Can you work these out from the drawing? Everything is in mm from the part's minimum corner. A direction names the side the tool comes from. Round coordinates to 2 decimals unless told otherwise and drop trailing zeros. Write each loop counter-clockwise with the first axis right and the second up, starting at its lowest first coordinate (ties: lowest second). Pieces come first, ordered by that corner, then holes. Notation, with made-up numbers: (-34.5, 43.5) -> (-27.5, 43.5) arc R29 ccw to (-27.5, 74.5) -> close; hole circle Ø11 at (35.25, 40.25). An arc over 180 degrees is marked (long way). Put each result on its own line as item: value. Start each with the question number.
1. Suppose I cut it at C-C (y = 6.5). Please give me the cut outline in (x, z), then the cut area to 3 significant figures.
2. Suppose I cut it at D-D (x = 11.5). Please give me the cut outline in (y, z).
3. Which directions (+Z, -Z, +X, -X, +Y, -Y) give clear straight access to the entire face, cutting with the end or side of a thin tool? Please do the marked faces 1 and 2.
4. I need wall thicknesses on probe 1 along Z at (x, y) = (16.7, 4.75); probe 2 along Z at (x, y) = (9, 17.25). Which ranges of each line are inside material? Lowest first, please. Write a range as from..to.
5. Suppose I cut it at A-A (y = 13.5). Please give me the cut outline in (x, z).
6. Suppose I cut it at B-B (z = 23.3). Please give me the cut outline in (x, y).
7. We'd pull the mould along X, two halves only. Please class the marked faces 3, 4, 5 and 6: +X half, -X half, draft (parallel to the pull), parting line (faces both ways), or undercut.
8. For pin 1 (6 mm diameter, centred on x = 16.5, z = 11.5, fed in from +Y); pin 2 (9 mm diameter, centred on x = 12, y = 12, fed in from +Z); pin 3 (4 mm diameter, centred on x = 6, z = 10, fed in from +Y), each with a flat end and sliding along its axis, tell me the tip position at first contact or that it passes through.
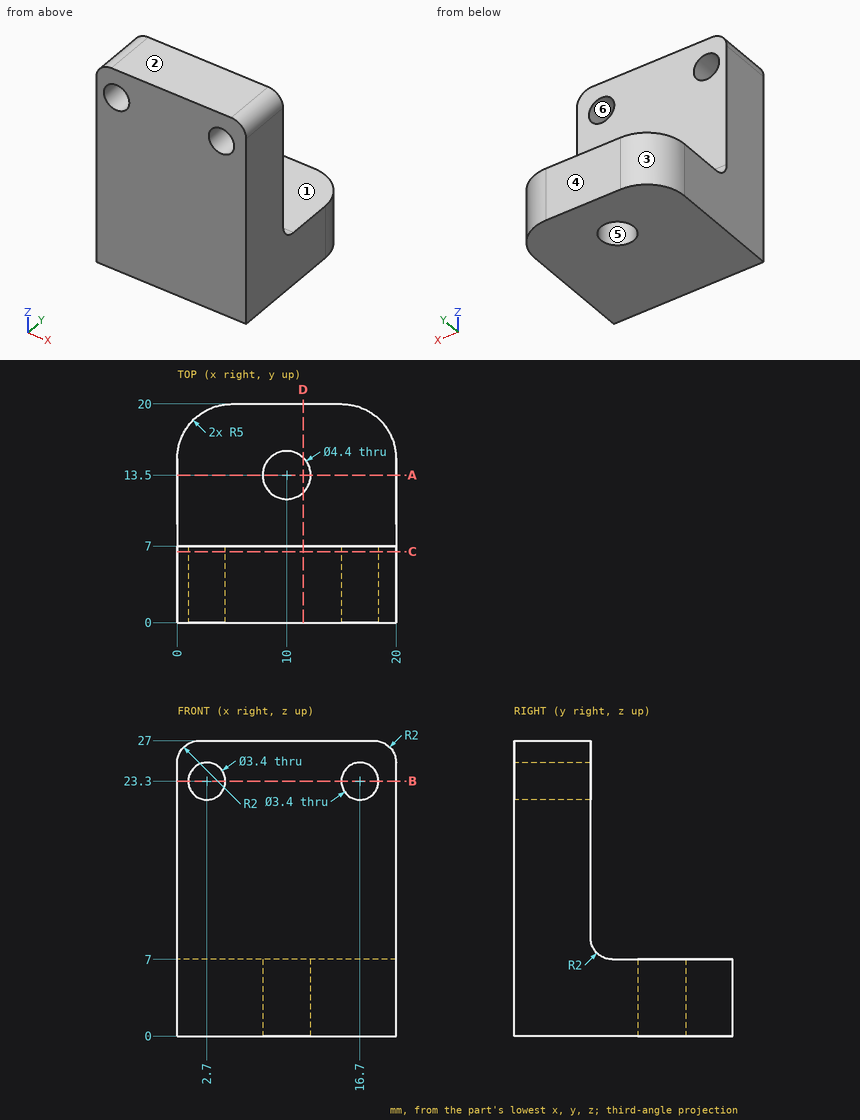
Verdict:
1. outline: (0, 0) -> (20, 0) -> (20, 25) arc R2 ccw to (18, 27) -> (2, 27) arc R2 ccw to (0, 25) -> close; hole circle Ø3.4 at (2.7, 23.3); hole circle Ø3.4 at (16.7, 23.3)
1. area: 520 mm^2
2. outline: (0, 0) -> (11.89, 0) -> (11.89, 7) -> (9, 7) arc R2 cw to (7, 9) -> (7, 27) -> (0, 27) -> close; (15.11, 0) -> (20, 0) -> (20, 7) -> (15.11, 7) -> close
3. face 1: +Z, +X, -X, +Y
3. face 2: +Z, +X, -X, +Y, -Y
4. probe 1: z = 0..21.6, 25..27
4. probe 2: z = 0..7
5. outline: (0, 0) -> (7.8, 0) -> (7.8, 7) -> (0, 7) -> close; (12.2, 0) -> (20, 0) -> (20, 7) -> (12.2, 7) -> close
6. outline: (0, 0) -> (1, 0) -> (1, 7) -> (0, 7) -> close; (4.4, 0) -> (15, 0) -> (15, 7) -> (4.4, 7) -> close; (18.4, 0) -> (20, 0) -> (20, 7) -> (18.4, 7) -> close
7. face 3: -X half
7. face 4: draft
7. face 5: undercut
7. face 6: undercut
8. pin 1: stops at y = 7.06
8. pin 2: stops at z = 7.68
8. pin 3: stops at y = 7.27
